Read the model definition and answer for the solid it produces. Units are mm, in the model's axes. Face numbers are marked on the shaded views. A direction names the side the tool comes from. Coordinates: 2 decimals unless noted, no trailing zeros. Order: outer loops, then holes, each group sorted by start corner. A loop starts at its lowest first (then second) coordinate and runs counter-clockwise, first axis right, second up.
```python
from build123d import *

# Parameters (mm, degrees)
SKETCH1_R           = 4.2
BOSS_EXTRUDE1_DEPTH = 70
SKETCH2_R           = 9.44
BOSS_EXTRUDE2_DEPTH = 86


with BuildPart() as part:
    # Sketch1 → Boss-Extrude1 (new body)
    with BuildSketch(Plane.XY):
        with BuildLine():
            Line((61, 0), (61, 92))
            Line((61, 92), (-189, 92))
            Line((-189, 92), (-189, 12))
            Line((-189, 12), (-59.808026217, 12))
            ThreePointArc((-59.808026217, 12), (-6.029527376, -60.701275107), (61, 0))
        make_face()
        with Locations((26.162950904, 26.162950904)):
            Circle(SKETCH1_R, mode=Mode.SUBTRACT)
        with Locations((26.162950904, -26.162950904)):
            Circle(SKETCH1_R, mode=Mode.SUBTRACT)
        with Locations((-26.162950904, -26.162950904)):
            Circle(SKETCH1_R, mode=Mode.SUBTRACT)
        with Locations((-26.162950904, 26.162950904)):
            Circle(SKETCH1_R, mode=Mode.SUBTRACT)
        with Locations((0, 63.5)):
            Circle(SKETCH1_R, mode=Mode.SUBTRACT)
    extrude(amount=-BOSS_EXTRUDE1_DEPTH)

    # Sketch2 → Boss-Extrude2 (add)
    with BuildSketch(Plane.XY):
        Circle(SKETCH2_R)
    extrude(amount=BOSS_EXTRUDE2_DEPTH)


solid = part.part
```
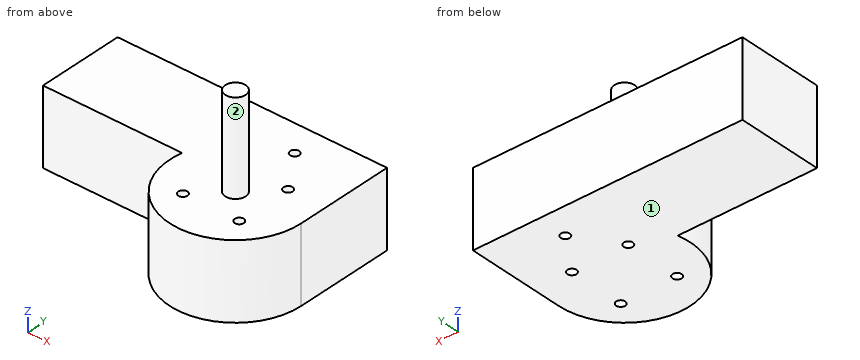
1) A cutting plane is placed at C-C, the plane z = 6. Determine the outline of the cut face in (x, y), and give its area (3 significant figures).
A:
outline: circle Ø18.88 at (0, 0)
area: 280 mm2
2) Which of the six approach directions +Z, -Z, +X, -X, +Y, -Y give full straight-line access (tool end or side, diameter ignored) to the marked faces 1 and 2?
A:
face 1: -Z, +X, -X, +Y, -Y
face 2: +Z
3) A cutting plane is placed at A-A, the plane y = 63.5. Determine the outline of the cut face in (x, z).
A:
outline: (-189, -70) - (-4.2, -70) - (-4.2, 0) - (-189, 0) - close; (4.2, -70) - (61, -70) - (61, 0) - (4.2, 0) - close
4) Flat-ended cylindrical pins translate along their axes: pin 1 Ø9.5 at (x, y) = (0, 63.5) entering from +Z; pin 2 Ø8 at (x, y) = (-63.5, -12.5) entering from -Z; pin 3 Ø3 at (y, z) = (-30, -24) entering from -X. Find the tip coordinate at first contact, or state that the pin passes through.
A:
pin 1: stops at z = 0
pin 2: stops at z = -70
pin 3: stops at x = -53.93
5) Straight lines are drawn through the part: line 1 (X direction, y = 25.5, z = -4); line 2 (Y direction, x = 27, z = -10); line 3 (Y direction, x = 0, z = -43). For each, find the intervals that lie inside material, in ascending order.
A:
line 1: x = -189 to -30.31, -22.02 to 22.02, 30.31 to 61
line 2: y = -54.7 to -30.28, -22.05 to 22.05, 30.28 to 92
line 3: y = -61 to 59.3, 67.7 to 92
6) A cutting plane is placed at D-D, the plane x = -173. Determine the outline of the cut face in (y, z), and give its area (3 significant figures).
A:
outline: (12, -70) - (92, -70) - (92, 0) - (12, 0) - close
area: 5,600 mm2
7) A cutting plane is placed at B-B, the plane x = 0. Determine the outline of the cut face in (y, z).
A:
outline: (-61, -70) - (59.3, -70) - (59.3, 0) - (9.44, 0) - (9.44, 86) - (-9.44, 86) - (-9.44, 0) - (-61, 0) - close; (67.7, -70) - (92, -70) - (92, 0) - (67.7, 0) - close
